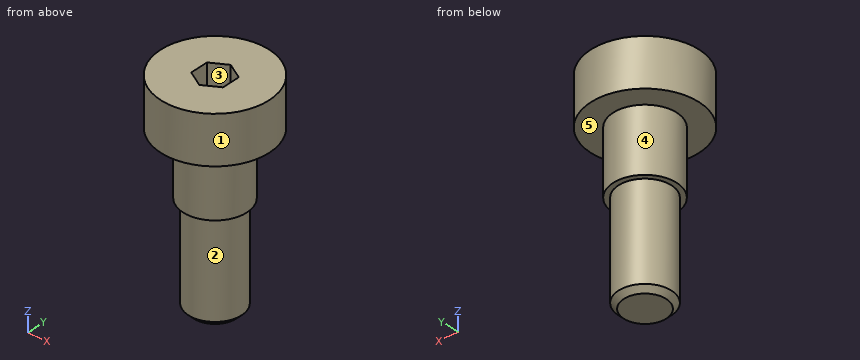
Solid Edge part; units mm, degrees
sketch "Sketch1" plane through (0, 0, 0) normal (0, 0, 1) x (1, 0, 0)
  circle A0 centre (0, 0) radius 5.11
extrude "Protrusion1" add sketch "Sketch1" along normal blind 4.5
sketch "Sketch2" plane through (0, 0, 4.5) normal (0, 0, 1) x (1, 0, 0)
  line L0 (0, -1.7321) -> (-1.5, -0.866)
  line L1 (-1.5, -0.866) -> (-1.5, 0.866)
  line L2 (-1.5, 0.866) -> (0, 1.7321)
  line L3 (0, 1.7321) -> (1.5, 0.866)
  line L4 (1.5, 0.866) -> (1.5, -0.866)
  line L5 (1.5, -0.866) -> (0, -1.7321)
extrude "Cutout1" cut sketch "Sketch2" against normal blind 2.25
sketch "Sketch3" plane through (0, 0, 0) normal (0, 0, -1) x (0, 1, 0)
  circle A0 centre (0, 0) radius 3
extrude "Protrusion2" add sketch "Sketch3" along normal blind 6
sketch "Sketch4" plane through (0, 0, -6) normal (0, 0, -1) x (0, 1, 0)
  circle A0 centre (0, 0) radius 2.5
extrude "Protrusion3" add sketch "Sketch4" along normal blind 9.5
chamfer "Chamfer1" distance 0.5 angle 45 1 edges at (0, -2.5, -15.5)
properties part number "24104609"
Model file for the job. Use its own axes, mm. Face numbers are marked on the shaded views. A direction names the side the tool comes from. Give positions to 0.01 mm unless a question says otherwise; leave off trailing zeros. Loops run counter-clockwise (first coordinate to the right, second up) from the corner with the lowest first, then second, coordinate; pieces in that order, holes last.
Item 1: Slice it at B-B (z = -2.25). Write the cut outline in (x, y).
Check values:
outline: circle Ø6 at (0, 0)
Item 2: Slice it at C-C (x = -3.25). Write the cut outline in (y, z).
Check values:
outline: (-3.94, 0) - (3.94, 0) - (3.94, 4.5) - (-3.94, 4.5) - close
Item 3: Mould opens along Y. For the marked faces 3, 4 and 5 say: +Y half, -Y half, draft (parallel to the pull), parting line (faces both ways), or undercut.
Check values:
face 3: undercut
face 4: parting line
face 5: draft
Item 4: Slice it at D-D (z = 0.75). Write the cut outline in (x, y).
Check values:
outline: circle Ø10.22 at (0, 0)
Item 5: Which spindle directions (+Z, -Z, +X, -X, +Y, -Y) get a long thin tool onto all of the face, cutting with end or side? Do the marked faces 1 and 2. Say none if no direction does.
Check values:
face 1: +Z, -Z
face 2: -Z
Item 6: Drill centre lines: line 1 along X through (y, z) = (0, -13.25); line 2 along Z through (x, y) = (2.25, 2.25); line 3 along Y through (x, z) = (2, -13.25). Where is each one in solid material? Low to high.
Check values:
line 1: x = -2.5 to 2.5
line 2: z = 0 to 4.5
line 3: y = -1.5 to 1.5
Item 7: Slice it at A-A (y = 0). Write the cut outline in (x, z), plus the area to 3 significant figures.
Check values:
outline: (-5.11, 0) - (-3, 0) - (-3, -6) - (-2.5, -6) - (-2.5, -15) - (-2, -15.5) - (2, -15.5) - (2.5, -15) - (2.5, -6) - (3, -6) - (3, 0) - (5.11, 0) - (5.11, 4.5) - (1.5, 4.5) - (1.5, 2.25) - (-1.5, 2.25) - (-1.5, 4.5) - (-5.11, 4.5) - close
area: 122 mm2
Item 8: Drop flat-ended pins along their axis: P1, Ø6, axis at x = -1.5, z = -7, coming from the +Y side; P2, Ø2, axis at x = 4, z = -12, coming from the +Y side; P3, Ø2, axis at y = 0.5, z = -10.5, coming from the +X side. Give the stop position or say it passes through.
Check values:
P1: stops at y = 3
P2: passes through
P3: stops at x = 2.5
